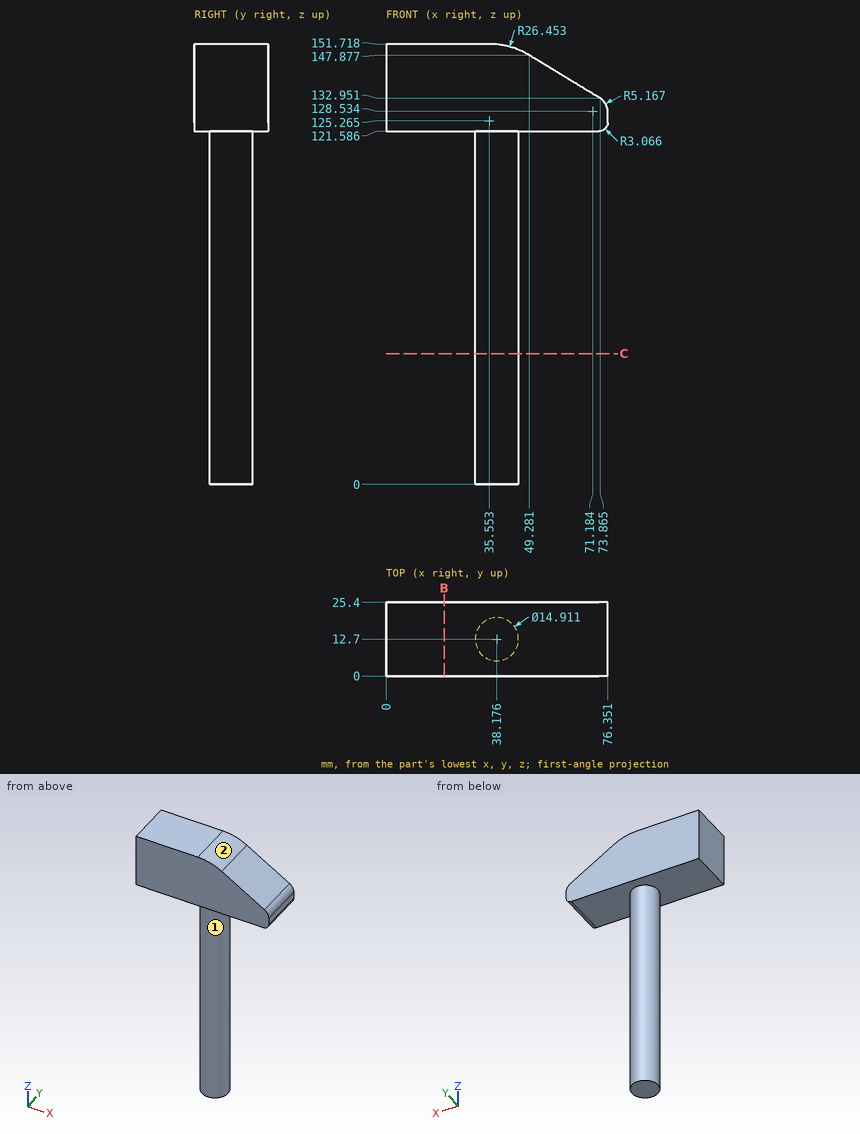
Here's the drawing with two shaded views (mm, measured from the low corner). I have some questions. A direction names the side the tool comes from. Coordinates: 2 decimals unless noted, no trailing zeros. Loops run counter-clockwise (first coordinate to the right, second up) from the corner with the lowest first, then second, coordinate; pieces in that order, holes last. Notation, with made-up numbers: (-17.5, 4.25) -> (41.5, 4.25) arc R15 ccw to (41.5, 15.25) -> close; hole circle Ø9 at (-29, -8). An arc over 180 degrees is marked (long way). Use one line per item in the form item = value. Start each with the question number.
(1) If we section it at B-B (x = 20): Please give me the cut outline in (y, z) (1 decimal).
(2) If we section it at C-C (z = 45): Please give me the cut outline in (x, y) (1 decimal).
(3) Please list where these lines run through material, in increasing order: line 1 along Z through (x, y) = (24, 18) (1 decimal); line 2 along Z through (x, y) = (47, 20.75) (1 decimal); line 3 along X through (y, z) = (17.5, 123).
(4) Will these pins go through, and if not, where does the flat tip stop? pin 1 (3 mm diameter, centred on x = 54, y = 16.5, fed in from +Z); pin 2 (5 mm diameter, centred on y = 5, z = 43, fed in from +X); pin 3 (8 mm diameter, centred on y = 4, z = 26.5, fed in from +X).
(5) On a 3-axis mill with a long thin cutter (end or side, diameter ignored), from which of +Z, -Z, +X, -X, +Y, -Y can I reach the whole of each face in a straight line? I mean the marked faces 1 and 2. Say none if no direction works.
Verdict:
q1.outline = (0, 121.6) -> (25.4, 121.6) -> (25.4, 151.7) -> (0, 151.7) -> close
q2.outline = circle Ø14.9 at (38.2, 12.7)
q3.line_1 = 121.6 to 151.7
q3.line_2 = 121.6 to 149.1
q3.line_3 = 0 to 75.87
q4.pin_1 = 145.92
q4.pin_2 = 43.52
q4.pin_3 = 43.96
q5.face_1 = -Z
q5.face_2 = +Z, +X, +Y, -Y
